The drawing under review shows one solid part. Ordinate dimensions are in mm from its lowest x, y, z. A direction names the side the tool comes from. Round coordinates to 2 decimals unless told otherwise and drop trailing zeros. Order: outer loops, then holes, each group sorted by start corner. A loop starts at its lowest first (then second) coordinate and runs counter-clockwise, first axis right, second up.
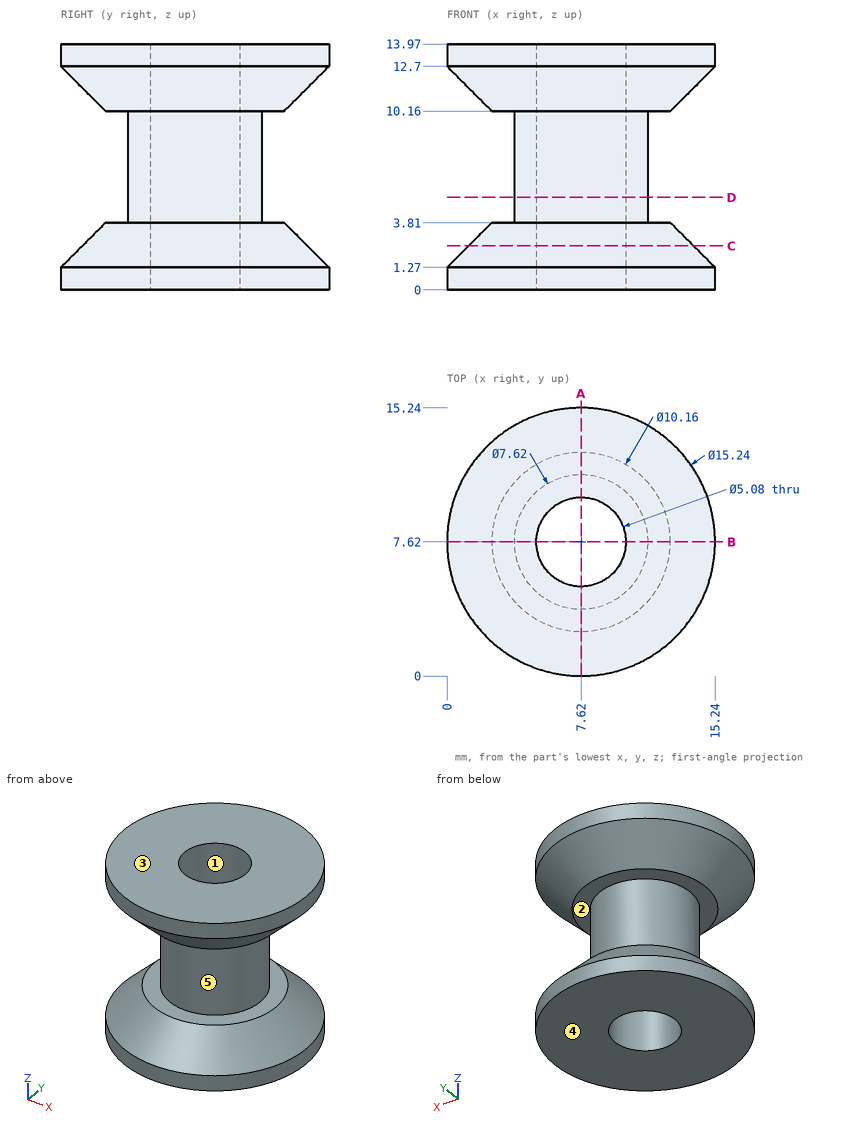
Q1. Mouldability with a two-part tool opening along Z and no side actions: class the marked faces 3, 4 and 5 as +Z half, -Z half, draft (parallel to the pull), parting line (faces both ways), or undercut.
Q2. Tool access review of the marked faces 1 and 2: name each direction out of +Z, -Z, +X, -X, +Y, -Y from which nothing blocks a thin tool from reaching the whole face with its end or side.
Q3. Take a section at C-C, the plane z = 2.5. State the section outline as (x, y) points, plus the area to 3 significant figures.
Q4. Take a section at D-D, the plane z = 5.25. State the section outline as (x, y) points, plus the area to 3 significant figures.
Q5. Clearance check with flat-ended pins moving along their axes: pin 1 (2 mm diameter, centred on x = 7.5, z = 2.5, fed in from +Y); pin 2 (4.5 mm diameter, centred on x = 7.62, y = 7.62, fed in from +Z); pin 3 (1 mm diameter, centred on y = 12, z = 10, fed in from +X); pin 4 (3 mm diameter, centred on x = 11, z = 9, fed in from -Y). State where each tip first meets the part, or that it passes through.
Q6. Wall thickness on line 1 (Y direction, x = 7.62, z = 6.25); line 2 (Z direction, x = 9.5, y = 12); line 3 (Y direction, x = 9.25, z = 5.25): over which ranges is each line inside the solid? List them lowest first.
Q7. Take a section at A-A, the plane x = 7.62. State the section outline as (y, z) points.
Working result:
1. face 3: +Z half
1. face 4: -Z half
1. face 5: undercut
2. face 1: +Z, -Z
2. face 2: none
3. outline: circle Ø12.78 at (7.62, 7.62); hole circle Ø5.08 at (7.62, 7.62)
3. area: 108 mm2
4. outline: circle Ø7.62 at (7.62, 7.62); hole circle Ø5.08 at (7.62, 7.62)
4. area: 25.3 mm2
5. pin 1: stops at y = 15.01
5. pin 2: passes through
5. pin 3: stops at x = 11.03
5. pin 4: stops at y = 3.11
6. line 1: y = 3.81 to 5.08, 10.16 to 11.43
6. line 2: z = 0 to 3.81, 10.16 to 13.97
6. line 3: y = 4.18 to 5.67, 9.57 to 11.06
7. outline: (0, 0) - (5.08, 0) - (5.08, 13.97) - (0, 13.97) - (0, 12.7) - (2.54, 10.16) - (3.81, 10.16) - (3.81, 3.81) - (2.54, 3.81) - (0, 1.27) - close; (10.16, 0) - (15.24, 0) - (15.24, 1.27) - (12.7, 3.81) - (11.43, 3.81) - (11.43, 10.16) - (12.7, 10.16) - (15.24, 12.7) - (15.24, 13.97) - (10.16, 13.97) - close
